```python
from build123d import *

# Parameters (mm, degrees)
ESQUISSE1_W             = 70
ESQUISSE1_H             = 30.03
BOSS_EXTRU_1_DEPTH      = 5
BOSS_EXTRU_2_START      = -5
ESQUISSE2_W             = 12
ESQUISSE2_H             = 5
BOSS_EXTRU_2_DEPTH      = 20
CONG_1_R                = 3
CONG_2_R                = 3
CONG_12_R               = 5
CONG_11_R               = 5
BOSS_EXTRU_5_DEPTH      = 70
CONG_13_R               = 10
CONG_14_R               = 5
ESQUISSE7_W             = 70
ESQUISSE7_H             = 5
BOSS_EXTRU_6_DEPTH      = 5
CONG_15_R               = 10
CONG_16_R               = 1
BOSS_EXTRU_7_START      = -2
BOSS_EXTRU_7_DEPTH      = 2
BOSS_EXTRU_8_START      = 4
BOSS_EXTRU_8_DEPTH      = 2
ESQUISSE11_R            = 2
ENL_V_MAT_EXTRU_1_DEPTH = 51.546043366
CONG_17_R               = 5


with BuildPart() as part:
    # Esquisse1 → Boss.-Extru.1 (new body)
    with BuildSketch(Plane.XY):
        Rectangle(ESQUISSE1_W, ESQUISSE1_H)
    extrude(amount=BOSS_EXTRU_1_DEPTH)

    # Esquisse2 → Boss.-Extru.2 (add)
    with BuildSketch(Plane.XY.offset(5).offset(BOSS_EXTRU_2_START)):
        with Locations((-26, 12.515)):
            Rectangle(ESQUISSE2_W, ESQUISSE2_H)
        with Locations((26, 12.515)):
            Rectangle(ESQUISSE2_W, ESQUISSE2_H)
    extrude(amount=-BOSS_EXTRU_2_DEPTH)

    # Congé1
    cong_1_edges = [part.edges().sort_by_distance(p)[0] for p in [
        (32, 12.515, 0),
    ]]
    fillet(cong_1_edges, radius=CONG_1_R - 0.0001)  # a hair under: the kernel refuses the full size

    # Congé2
    cong_2_edges = [part.edges().sort_by_distance(p)[0] for p in [
        (-32, 12.515, 0),
    ]]
    fillet(cong_2_edges, radius=CONG_2_R - 0.0001)  # a hair under: the kernel refuses the full size

    # Congé12
    cong_12_edges = [part.edges().sort_by_distance(p)[0] for p in [
        (-20, 12.515, 0),
    ]]
    fillet(cong_12_edges, radius=CONG_12_R)

    # Congé11
    cong_11_edges = [part.edges().sort_by_distance(p)[0] for p in [
        (20, 12.515, 0),
    ]]
    fillet(cong_11_edges, radius=CONG_11_R)

    # Esquisse6 → Boss.-Extru.5 (add, through all)
    with BuildSketch(Plane(origin=(35, 0, 0), x_dir=(0, 0, -1), z_dir=(1, 0, 0))):
        Polygon((-5, 15.015), (-25, 15.015), (-25, 36.565), (-20, 36.565), (-20, 21.515), (-5, 21.515), (0, 21.515), (0, 15.015), align=None)
    extrude(amount=-BOSS_EXTRU_5_DEPTH)

    # Congé13
    cong_13_edges = [part.edges().sort_by_distance(p)[0] for p in [
        (0, 15.015, 25),
    ]]
    fillet(cong_13_edges, radius=CONG_13_R)

    # Congé14
    cong_14_edges = [part.edges().sort_by_distance(p)[0] for p in [
        (0, 36.565, 25),
    ]]
    fillet(cong_14_edges, radius=CONG_14_R - 0.0001)  # a hair under: the kernel refuses the full size

    # Esquisse7 → Boss.-Extru.6 (add)
    with BuildSketch(Plane(origin=(0, 0, 20), x_dir=(-1, 0, 0), z_dir=(0, 0, -1))):
        with Locations((0, 34.065)):
            Rectangle(ESQUISSE7_W, ESQUISSE7_H)
    extrude(amount=BOSS_EXTRU_6_DEPTH)

    # Congé15
    cong_15_edges = [part.edges().sort_by_distance(p)[0] for p in [
        (0, 15.015, 5),
    ]]
    fillet(cong_15_edges, radius=CONG_15_R - 0.0001)  # a hair under: the kernel refuses the full size

    # Congé16
    cong_16_edges = [part.edges().sort_by_distance(p)[0] for p in [
        (0, 21.515, 0),
    ]]
    fillet(cong_16_edges, radius=CONG_16_R)

    # Esquisse8 → Boss.-Extru.7 (add)
    with BuildSketch(Plane(origin=(32, 0, 0), x_dir=(0, 0, -1), z_dir=(1, 0, 0)).offset(BOSS_EXTRU_7_START)):
        Polygon((1, 15.015), (0, 20.515), (0, 15.009679375), align=None)
    boss_extru_7 = extrude(amount=-BOSS_EXTRU_7_DEPTH)

    # Esquisse9 → Boss.-Extru.8 (add)
    with BuildSketch(Plane.ZY.offset(-28).offset(BOSS_EXTRU_8_START)):
        Polygon((0, 20.515), (-1, 15.015), (0, 15.015), align=None)
    boss_extru_8 = extrude(amount=BOSS_EXTRU_8_DEPTH)

    # Symétrie3: Boss.-Extru.7, Boss.-Extru.8 across plane
    add(boss_extru_7.mirror(Plane(origin=(0, 0, 0), x_dir=(0, 0, 1), z_dir=(1, 0, 0))))
    add(boss_extru_8.mirror(Plane(origin=(0, 0, 0), x_dir=(0, 0, 1), z_dir=(1, 0, 0))))

    # Esquisse11 → Enlèv. mat.-Extru.1 (cut, through all)
    with BuildSketch(Plane.XZ.offset(-10.015)):
        with Locations((25.2, -15)):
            Circle(ESQUISSE11_R)
        with Locations((25.2, -5)):
            Circle(ESQUISSE11_R)
        with Locations((-25.2, -15)):
            Circle(ESQUISSE11_R)
        with Locations((-25.2, -5)):
            Circle(ESQUISSE11_R)
    extrude(amount=-ENL_V_MAT_EXTRU_1_DEPTH, mode=Mode.SUBTRACT)

    # Congé17
    cong_17_edges = [part.edges().sort_by_distance(p)[0] for p in [
        (-32, 12.515, -20),
        (32, 12.515, -20),
    ]]
    fillet(cong_17_edges, radius=CONG_17_R)


solid = part.part
```
Geometry check sheet. Reference: the model listing, model coordinates, mm. A direction names the side the tool comes from. Coordinates: 2 decimals unless noted, no trailing zeros. Loops run counter-clockwise (first coordinate to the right, second up) from the corner with the lowest first, then second, coordinate; pieces in that order, holes last. Notation, with made-up numbers: (9, 12.5) - (39, 12.5) arc R17 cw to (39, 42.5) - close; hole circle Ø1 at (38, 86). An arc over 180 degrees is marked (long way). One line per item, written item: value. Start each with the question number.
(1) Material ranges on line 1 (Z direction, x = -25.2, y = 12.35); line 2 (Z direction, x = -25, y = 14); line 3 (Y direction, x = 19.5, z = 4) (3 decimals), recorded low to high. Write a range as [from, to].
(2) Mould release check, pull along Z, two halves, no side actions. Record for faces 5 (the flat face through (25, 10.015, -10)), 6 (the cylindrical face through (-27.198, 12.48, -14.912)), 7 (the flat face through (-23.014, 17.804, -0.493)): released by +Z, released by -Z, zero draft, split by the parting line, or undercut.
(3) Cross-section at C-C on y = -3.5. Enter the section's corners in (x, z), plus the area to 3 significant figures.
(4) Depth check by flat-ended pin: P1, Ø16, axis at x = -25, z = -13.5, coming from the -Y side (3 decimals); P2, Ø4.5, axis at x = -26, y = 18.5, coming from the -Z side; P3, Ø2, axis at x = 0, y = -5.5, coming from the +Z side. Enter the tip coordinate at first touch or a pass-through.
(5) Tool access check on faces 1 (the cylindrical face through (-19, 13, -2)), 2 (the flat face through (0, 21.515, 10)), 3 (the flat face through (0, -5, 5)), 4 (the flat face through (-32, 12, -9)). Record the directions out of +Z, -Z, +X, -X, +Y, -Y that give a thin tool (end or side, any length) a straight path to the whole face; none if there is none.
(6) Cross-section at A-A on x = 25.2. Count the separate pieces of the cut face and the enclosed holes in it, plus the area to 3 significant figures.
(7) Cross-section at D-D on z = 11. Enter the section's corners in (x, y) (3 decimals), plus the area to 3 significant figures.
Results below:
1. line 1: z = [-20, -17], [-13, -7], [-3, 8.2]
1. line 2: z = [-20, -16.99], [-13.01, -6.99], [-3.01, 10.61]
1. line 3: y = [-15.015, 21.515]
2. face 5: zero draft
2. face 6: undercut
2. face 7: released by -Z
3. outline: (-35, 0) - (35, 0) - (35, 5) - (-35, 5) - close
3. area: 350 mm2
4. P1: stops at y = 10.015
4. P2: stops at z = -0.55
4. P3: stops at z = 5
5. face 1: -Z, +Y, -Y
5. face 2: -Z, +X, -X
5. face 3: +Z, +X, -X, -Y
5. face 4: -Z, -X, +Y, -Y
6. separate pieces: 3
6. enclosed holes: 0
6. area: 467 mm2
7. outline: (-35, 14.18) - (35, 14.18) - (35, 21.515) - (-35, 21.515) - close
7. area: 513 mm2
